```python
from build123d import *

# Parameters (mm, degrees)
BOSS_EXTRUDE1_START = -1
BOSS_EXTRUDE1_DEPTH = 32
CIRPATTERN3_COUNT   = 12
BOSS_EXTRUDE2_START = -2
SKETCH5_R           = 0.75
BOSS_EXTRUDE2_DEPTH = 100


with BuildPart() as part:
    # Sketch3 → Boss-Extrude1 (new body)
    with BuildSketch(Plane(origin=(0, 0, 0), x_dir=(0, 0, -1), z_dir=(1, 0, 0)).offset(BOSS_EXTRUDE1_START)):
        with BuildLine():
            Line((-2, 22.226110771), (-2, 12.821942467))
            Line((-2, 12.821942467), (-4.678920426, 12.104127903))
            Line((-4.678920426, 12.104127903), (-9.381004578, 20.248376555))
            ThreePointArc((-9.381004578, 20.248376555), (-9.496151336, 21.498457721), (-8.620764237, 22.398268325))
            ThreePointArc((-8.620764237, 22.398268325), (-6.211657082, 23.182219831), (-3.733333333, 23.707851489))
            ThreePointArc((-3.733333333, 23.707851489), (-2.525320566, 23.366286196), (-2, 22.226110771))
        make_face()
    boss_extrude1 = extrude(amount=BOSS_EXTRUDE1_DEPTH)

    # Sketch4 → Revolve1 (revolve)
    with BuildSketch(Plane.XY):
        with BuildLine():
            Line((-1, 24.5), (-14, 24.5))
            ThreePointArc((-14, 24.5), (-15.414213562, 23.914213562), (-16, 22.5))
            Line((-16, 22.5), (-16, 14.5))
            ThreePointArc((-16, 14.5), (-15.414213562, 13.085786438), (-14, 12.5))
            Line((-14, 12.5), (-1, 12.5))
            Line((-1, 12.5), (-1, 24.5))
        make_face()
        with BuildLine():
            Line((31, 24.5), (39, 24.5))
            ThreePointArc((39, 24.5), (40.414213562, 23.914213562), (41, 22.5))
            Line((41, 22.5), (41, 14.5))
            ThreePointArc((41, 14.5), (40.414213562, 13.085786438), (39, 12.5))
            Line((39, 12.5), (31, 12.5))
            Line((31, 12.5), (31, 24.5))
        make_face()
    revolve(axis=Axis((-2, 0, 0), (1, 0, 0)))

    # CirPattern3: Boss-Extrude1 ×12 about axis
    cirpattern3_axis = Axis((0, 0, 0), (1, 0, 0))
    for i in range(1, CIRPATTERN3_COUNT):
        add(boss_extrude1.rotate(cirpattern3_axis, i * 360 / CIRPATTERN3_COUNT))

    # Sketch5 → Boss-Extrude2 (add)
    with BuildSketch(Plane(origin=(0, 0, 0), x_dir=(0, 0, -1), z_dir=(1, 0, 0)).offset(BOSS_EXTRUDE2_START)):
        with Locations((-1.3, 19)):
            Circle(SKETCH5_R)
        with Locations((0, 21.25166605)):
            Circle(SKETCH5_R)
        with Locations((1.3, 19)):
            Circle(SKETCH5_R)
    extrude(amount=-BOSS_EXTRUDE2_DEPTH)


solid = part.part
```
Input: part model. Units: mm. Frame: model coordinates. A direction names the side the tool comes from. Round coordinates to 2 decimals unless told otherwise and drop trailing zeros. Loops run counter-clockwise (first coordinate to the right, second up) from the corner with the lowest first, then second, coordinate; pieces in that order, holes last. Notation, with made-up numbers: M 57,28.25 L 79,28.25 A26 cw 79,45.25 Z; hole C -30.75,-9.75 d6. An arc over 180 degrees is marked long. Answer in a Markdown table with one row per item. Add a question column.
1. Section B-B (x = 12). Give the number of separate pieces and of enclosed holes in the cut face, and give its area (3 significant figures).
2. Set-up query: faces 1 (the face through (-1, -1.7, 12.8)), 2 (the face through (15, 2, 17)), 3 (the face through (14.776, -16.945, -16.996)), 4 (the face through (15, -17, 2)). Return all of +Z, -Z, +X, -X, +Y, -Y with unobstructed straight access to the full face (end or side cutting, diameter ignored); none if empty.
3. Section A-A (y = 0). Output: boundary loops of the cut face in (x, z), and give its area (3 significant figures).
4. Mould query, pull axis X, two halves, no side actions, for faces 5 (the face through (15, -2, -17)), 6 (the face through (34.944, 11.923, 3.755)), 7 (the face through (-16, 0, -15)). Classes: released by +X, released by -X, zero draft, split by the parting line, or undercut.
5. Contact query for flat-ended pins moving along their axis: pin 1 (10.5 mm diameter, centred on x = 18.5, y = 16.5, fed in from +Z); pin 2 (8 mm diameter, centred on x = -3, y = -13.5, fed in from +Z); pin 3 (4.5 mm diameter, centred on x = 14, y = -18.5, fed in from +Z). Output: stop coordinate, or through.
6. Section C-C (x = -63). Output: boundary loops of the cut face in (y, z).
7. Ray query, probe 1 along Z at (x, y) = (35.5, 0); probe 2 along X at (y, z) = (16.5, -1); probe 3 along Z at (x, y) = (26.5, -9). Return the intervals inside material, ascending.
Values follow:
| question | item | result |
|---|---|---|
| 1 | separate pieces | 12 |
| 1 | enclosed holes | 0 |
| 1 | area | 736 mm^2 |
| 2 | face 1 | none |
| 2 | face 2 | +Z, -Z |
| 2 | face 3 | -Z, -Y |
| 2 | face 4 | +Y, -Y |
| 3 | outline | M -16,-22.5 A2 ccw -14,-24.5 L -1,-24.5 L -1,-12.5 L -14,-12.5 A2 ccw -16,-14.5 Z; M -16,14.5 A2 ccw -14,12.5 L -1,12.5 L -1,24.5 L -14,24.5 A2 ccw -16,22.5 Z; M 31,-24.5 L 39,-24.5 A2 ccw 41,-22.5 L 41,-14.5 A2 ccw 39,-12.5 L 31,-12.5 Z; M 31,12.5 L 39,12.5 A2 ccw 41,14.5 L 41,22.5 A2 ccw 39,24.5 L 31,24.5 Z |
| 3 | area | 593 mm^2 |
| 4 | face 5 | undercut |
| 4 | face 6 | zero draft |
| 4 | face 7 | released by -X |
| 5 | pin 1 | z = 19 |
| 5 | pin 2 | z = 22.58 |
| 5 | pin 3 | z = 17.66 |
| 6 | outline | C 19,-1.3 d1.5; C 19,1.3 d1.5; C 21.25,0 d1.5 |
| 7 | probe 1 | -24.5 to -12.5, 12.5 to 24.5 |
| 7 | probe 2 | -16 to -1, 31 to 41 |
| 7 | probe 3 | -22.18 to -19.59, -11.59 to -9.25, 9.25 to 11.59, 19.59 to 22.18 |
